Study the drawing (mm; zero at the part's minimum x, y, z) and answer. A direction names the side the tool comes from. Round coordinates to 2 decimals unless told otherwise and drop trailing zeros. Write each loop counter-clockwise with the first axis right and the second up, starting at its lowest first coordinate (ties: lowest second). Pieces come first, ordered by that corner, then holes. Notation, with made-up numbers: (-7, 74) - (38, 74) arc R22 cw to (38, 89) - close; hole circle Ø5 at (16.25, 3). An arc over 180 degrees is marked (long way). Use one line per item in the form item = value. Start each with the question number.
1) The part is cut by section A-A, the plane z = 10. Give the vertices of the cut face in (x, y).
2) The part is cut by section D-D, the plane x = 16.75. Give the vertices of the cut face in (y, z), plus the area to 3 significant figures.
3) The part is cut by section B-B, the plane x = 7.25. Give the vertices of the cut face in (y, z), plus the area to 3 significant figures.
4) For the marked faces 1, 2 and 3, determine the directions among +Z, -Z, +X, -X, +Y, -Y from which every point of the face is accessible in a straight line to the end or side of a thin tool.
5) Consider line 1 along Y through (x, z) = (14.75, 12.75); line 2 along X through (y, z) = (47, 9.75). Determine where each line is inside the solid, lowest interval first. Write a range as from..to.
6) Each of these flat-tipped pins is pushed along its axis until it touches: pin 1 (1 mm diameter, centred on x = 13.5, y = 66.5, fed in from +Z); pin 2 (8 mm diameter, centred on x = 4.5, y = 67, fed in from +Z); pin 3 (3 mm diameter, centred on y = 52.5, z = 4, fed in from +X). Where does it stop, or does it pass through?
7) The part is cut by section C-C, the plane y = 39.5. Give the vertices of the cut face in (x, z), plus the area to 3 significant figures.
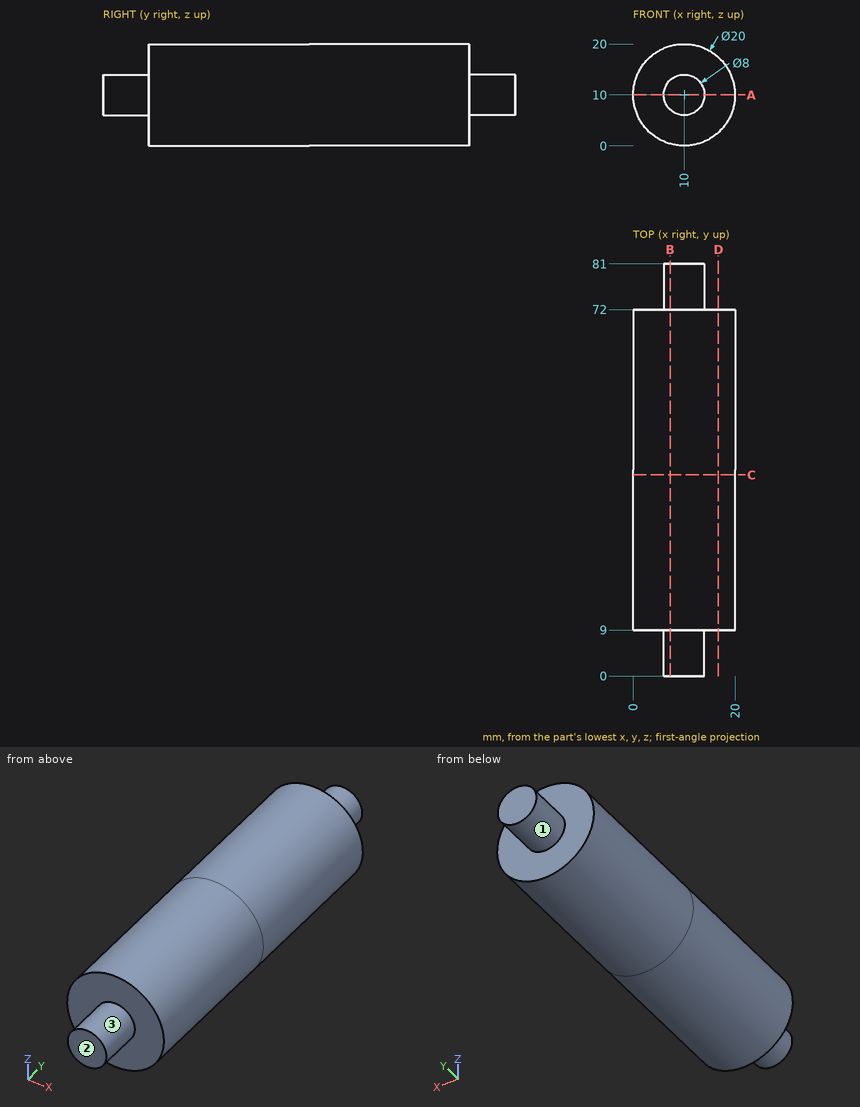
Geometry results:
q1.outline = (0, 9) - (6, 9) - (6, 0) - (14, 0) - (14, 9) - (20, 9) - (20, 72) - (14, 72) - (14, 81) - (6, 81) - (6, 72) - (0, 72) - close
q2.outline = (9, 2.62) - (72, 2.62) - (72, 17.38) - (9, 17.38) - close
q2.area = 930 mm2
q3.outline = (0, 7.1) - (9, 7.1) - (9, 0.39) - (72, 0.39) - (72, 7.1) - (81, 7.1) - (81, 12.9) - (72, 12.9) - (72, 19.61) - (9, 19.61) - (9, 12.9) - (0, 12.9) - close
q3.area = 1,320 mm2
q4.face_1 = +Y
q4.face_2 = +Z, -Z, +X, -X, -Y
q4.face_3 = -Y
q5.line_1 = 9..72
q5.line_2 = 0..20
q6.pin_1 = 19.54
q6.pin_2 = 19.89
q6.pin_3 = 18.93
q7.outline = circle Ø20 at (10, 10)
q7.area = 314 mm2
